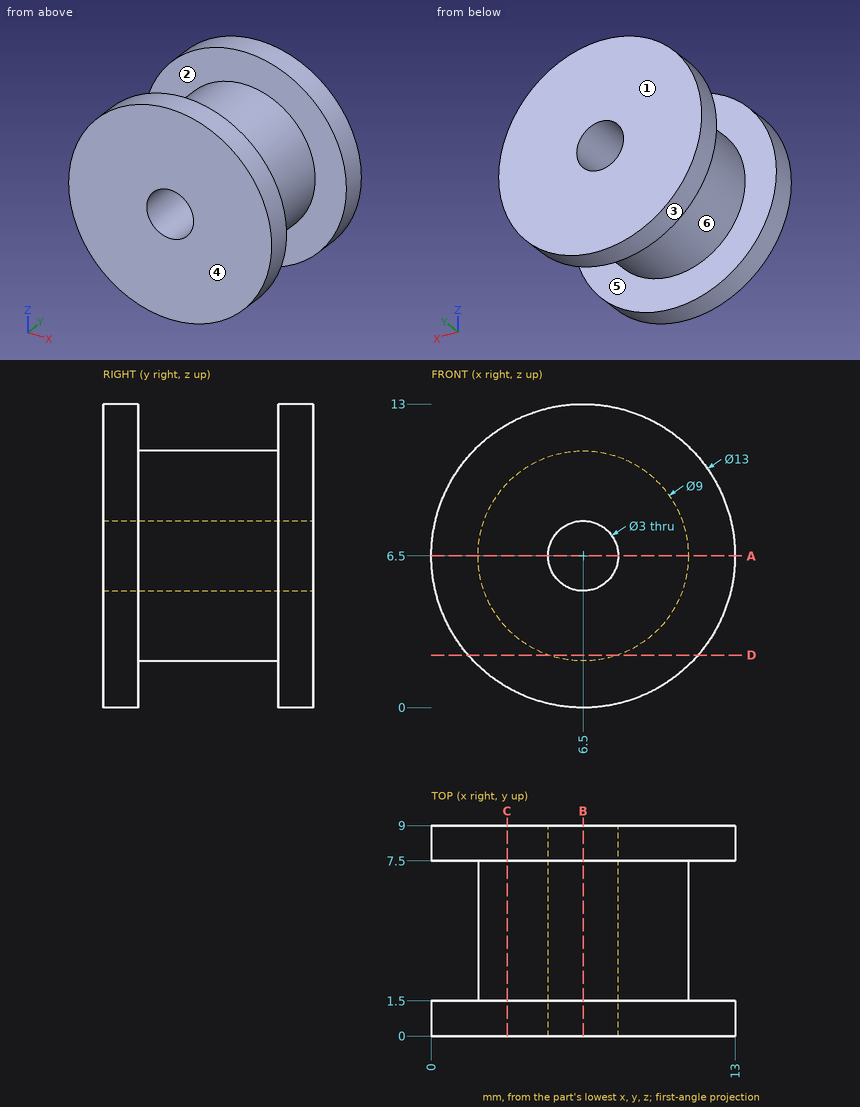
Study the drawing (mm; zero at the part's minimum x, y, z) and answer. A direction names the side the tool comes from. Give positions to 0.01 mm unless a question says otherwise; leave off trailing zeros. Loops run counter-clockwise (first coordinate to the right, second up) from the corner with the lowest first, then second, coordinate; pieces in that order, holes last. Notation, with made-up numbers: M 12,7.25 L 29,7.25 A20 ccw 29,41.25 Z; hole C 65,58 d7. An arc over 180 degrees is marked long. One line per item, written item: value. Start each with the question number.
1. Find section B-B (x = 6.5). Give the vertices of the cut face in (y, z).
2. Which of the six approach directions +Z, -Z, +X, -X, +Y, -Y give full straight-line access (tool end or side, diameter ignored) to the marked faces 1 and 2?
3. Find section C-C (x = 3.25). Give the vertices of the cut face in (y, z), and give its area (3 significant figures).
4. Find section A-A (z = 6.5). Give the vertices of the cut face in (x, y), and give its area (3 significant figures).
5. Find section D-D (z = 2.25). Give the vertices of the cut face in (x, y), and give its area (3 significant figures).
6. Determine the mould class of the marked faces 3, 4, 5 and 6 for opening direction Y: released by +Y, released by -Y, zero draft, split by the parting line, or undercut.
7. Each of these flat-tipped pins is pushed along its axis until it touches: P1, Ø1.5, axis at y = 7.5, z = 10, coming from the -X side; P2, Ø5, axis at x = 10, y = 3.5, coming from the -Z side; P3, Ø1.8, axis at x = 6.5, z = 6.5, coming from the +Y side; P4, Ø1, axis at x = 8.5, z = 4.5, coming from the -Y side. Where does it stop, or does it pass through?
8. Find the intervals of material crossed by probe 1 along Z at (x, y) = (6.5, 4); probe 2 along Y at (x, z) = (9, 2.5), in increasing order.
Reported:
1. outline: M 0,0 L 1.5,0 L 1.5,2 L 7.5,2 L 7.5,0 L 9,0 L 9,5 L 0,5 Z; M 0,8 L 9,8 L 9,13 L 7.5,13 L 7.5,11 L 1.5,11 L 1.5,13 L 0,13 Z
2. face 1: +Z, -Z, +X, -X, +Y
2. face 2: none
3. outline: M 0,0.87 L 1.5,0.87 L 1.5,3.39 L 7.5,3.39 L 7.5,0.87 L 9,0.87 L 9,12.13 L 7.5,12.13 L 7.5,9.61 L 1.5,9.61 L 1.5,12.13 L 0,12.13 Z
3. area: 71.1 mm²
4. outline: M 0,0 L 5,0 L 5,9 L 0,9 L 0,7.5 L 2,7.5 L 2,1.5 L 0,1.5 Z; M 8,0 L 13,0 L 13,1.5 L 11,1.5 L 11,7.5 L 13,7.5 L 13,9 L 8,9 Z
4. area: 66.0 mm²
5. outline: M 1.58,0 L 11.42,0 L 11.42,1.5 L 7.98,1.5 L 7.98,7.5 L 11.42,7.5 L 11.42,9 L 1.58,9 L 1.58,7.5 L 5.02,7.5 L 5.02,1.5 L 1.58,1.5 Z
5. area: 47.3 mm²
6. face 3: zero draft
6. face 4: released by -Y
6. face 5: undercut
6. face 6: undercut
7. P1: stops at x = 0.61
7. P2: stops at z = 0.32
7. P3: passes through
7. P4: stops at y = 0
8. probe 1: z = 2 to 5, 8 to 11
8. probe 2: y = 0 to 1.5, 7.5 to 9
